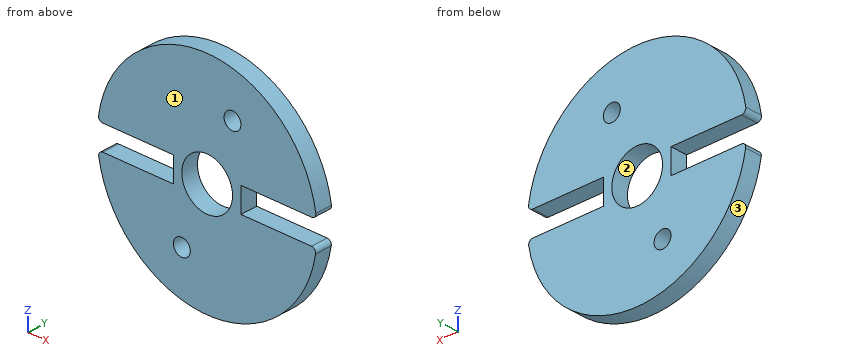
```python
from build123d import *

# Parameters (mm, degrees)
SKETCH1_R           = 1
SKETCH1_R_2         = 3
BOSS_EXTRUDE1_DEPTH = 2


with BuildPart() as part:
    # Sketch1 → Boss-Extrude1 (new body)
    with BuildSketch(Plane(origin=(0, 0, 0), x_dir=(1, 0, 0), z_dir=(0, 1, 0))):
        with BuildLine():
            Line((-12.338962679, 1.5), (-4, 1.5))
            Line((-4, 1.5), (-4, -1.388047838))
            Line((-4, -1.388047838), (-12.356588338, -1.388047838))
            ThreePointArc((-12.356588338, -1.388047838), (-12.735904141, -1.562287924), (-12.850851872, -1.963569752))
            ThreePointArc((-12.850851872, -1.963569752), (0, -13), (12.850851872, -1.963569752))
            ThreePointArc((12.850851872, -1.963569752), (12.735904141, -1.562287924), (12.356588338, -1.388047838))
            Line((12.356588338, -1.388047838), (4, -1.388047838))
            Line((4, -1.388047838), (4, 1.5))
            Line((4, 1.5), (12.338962679, 1.5))
            ThreePointArc((12.338962679, 1.5), (12.719751335, 1.675962965), (12.832521186, 2.08))
            ThreePointArc((12.832521186, 2.08), (0, 13), (-12.832521186, 2.08))
            ThreePointArc((-12.832521186, 2.08), (-12.719751335, 1.675962965), (-12.338962679, 1.5))
        make_face()
        with Locations((-2.996852747, 7.417470837)):
            Circle(SKETCH1_R, mode=Mode.SUBTRACT)
        with Locations((2.996852747, -7.417470837)):
            Circle(SKETCH1_R, mode=Mode.SUBTRACT)
        Circle(SKETCH1_R_2, mode=Mode.SUBTRACT)
    extrude(amount=BOSS_EXTRUDE1_DEPTH)


solid = part.part
```
Read the model definition and answer for the solid it produces. Units are mm, in the model's axes. Face numbers are marked on the shaded views. Round coordinates to 2 decimals unless told otherwise and drop trailing zeros. Write each loop counter-clockwise with the first axis right and the second up, starting at its lowest first coordinate (ties: lowest second). Pieces come first, ordered by that corner, then holes. Notation, with made-up numbers: (39, 11.25) -> (47, 11.25) arc R20 ccw to (47, 33.25) -> close; hole circle Ø11 at (2.5, 54.25). An arc over 180 degrees is marked (long way). Answer in a Markdown table with one row per item. Add a question column.
1) Consider line 1 (X direction, y = 0.65, z = 0); line 2 (X direction, y = 1.85, z = 7.5); line 3 (Z direction, x = 8, y = 0.8). Determine where each line is inside the solid, lowest interval first.
2) Find section D-D, the plane z = -5.5. Determine the outline of the cut face in (x, y), and give its area (3 significant figures).
3) Find section C-C, the plane y = 1.5. Determine the outline of the cut face in (x, z), and give its area (3 significant figures).
4) Determine the mould class of the marked faces 1, 2 and 3 for opening direction Z: pulls with the +Z half, pulls with the -Z half, needs draft (parallel to the pull), parting line crosses it, or undercut.
5) Given P1, Ø0.6, axis at y = 1.5, z = 0, coming from the -X side; P2, Ø1, axis at x = -8.5, y = 1.5, coming from the +Z side; P3, Ø1, axis at x = 6.5, y = 1.5, coming from the -Z side, each flat-ended and moving along its own axis, determine where each tip first touches the part or whether it passes through.
6) Find section A-A, the plane x = 0. Determine the outline of the cut face in (y, z).
7) Find section B-B, the plane z = 0. Determine the outline of the cut face in (x, y), and give its area (3 significant figures).
Findings below:
| question | item | result |
|---|---|---|
| 1 | line 1 | -4 to -3, 3 to 4 |
| 1 | line 2 | -10.62 to 2, 3.99 to 10.62 |
| 1 | line 3 | -10.25 to -1.5, 1.39 to 10.25 |
| 2 | outline | (-11.78, 0) -> (11.78, 0) -> (11.78, 2) -> (-11.78, 2) -> close |
| 2 | area | 47.1 mm² |
| 3 | outline | (-12.85, 1.96) arc R0.5 ccw to (-12.36, 1.39) -> (-4, 1.39) -> (-4, -1.5) -> (-12.34, -1.5) arc R0.5 ccw to (-12.83, -2.08) arc R13 ccw to (12.83, -2.08) arc R0.5 ccw to (12.34, -1.5) -> (4, -1.5) -> (4, 1.39) -> (12.36, 1.39) arc R0.5 ccw to (12.85, 1.96) arc R13 ccw to start; hole circle Ø2 at (-3, -7.42); hole circle Ø6 at (0, 0); hole circle Ø2 at (3, 7.42) |
| 3 | area | 444 mm² |
| 4 | face 1 | needs draft |
| 4 | face 2 | undercut |
| 4 | face 3 | pulls with the -Z half |
| 5 | P1 | x = -4 |
| 5 | P2 | z = 10.25 |
| 5 | P3 | z = -11.53 |
| 6 | outline | (0, -13) -> (2, -13) -> (2, -3) -> (0, -3) -> close; (0, 3) -> (2, 3) -> (2, 13) -> (0, 13) -> close |
| 7 | outline | (-4, 0) -> (-3, 0) -> (-3, 2) -> (-4, 2) -> close; (3, 0) -> (4, 0) -> (4, 2) -> (3, 2) -> close |
| 7 | area | 4.00 mm² |
